Work out the finished part from the listing and answer in its coordinate system (mm). A direction names the side the tool comes from. Round coordinates to 2 decimals unless told otherwise and drop trailing zeros. Loops run counter-clockwise (first coordinate to the right, second up) from the corner with the lowest first, then second, coordinate; pieces in that order, holes last.
Autodesk Inventor part; units mm, degrees
ref_plane "YZ Plane" through (0, 0, 0) normal (1, 0, 0) x (0, 1, 0)
ref_plane "XZ Plane" through (0, 0, 0) normal (0, 1, 0) x (-1, 0, 0)
ref_plane "XY Plane" through (0, 0, 0) normal (0, 0, 1) x (1, 0, 0)
sketch "Szkic1" plane through (0, 0, 0) normal (0, 0, 1) x (1, 0, 0)
  line L0 (0, 0) -> (20, 0)
  line L1 (0, 0) -> (-20, 0)
  line L2 (-20, 0) -> (-20, 20)
  line L3 (-20, 0) -> (0, 0) construction
  line L4 (-20, 20) -> (20, 20)
  line L5 (20, 20) -> (20, 0)
  line L6 (-20, 0) -> (-20, 88)
  line L7 (-20, 88) -> (20, 88)
  line L8 (20, 88) -> (20, 20)
  line L9 (20, 88) -> (20, 93)
  line L10 (20, 93) -> (-20, 93)
  line L11 (-20, 93) -> (-20, 88)
  line L12 (0, 93) -> (35, 93)
  line L13 (35, 93) -> (40, 93)
  line L14 (0, 93) -> (-35, 93)
  line L15 (-35, 93) -> (-40, 93)
  line L16 (-40, 93) -> (-40, 103)
  line L17 (-40, 103) -> (40, 103)
  line L18 (40, 103) -> (40, 93)
  line L19 (-35, 93) -> (-35, 103)
  line L20 (35, 93) -> (35, 103)
  circle A0 centre (-35, 103) radius 1.5
  circle A1 centre (-35, 93) radius 1.5
  circle A2 centre (35, 103) radius 1.5
  circle A3 centre (35, 93) radius 1.5
  line L21 (40, 93) -> (40, 83)
  line L22 (40, 83) -> (20, 83)
  line L23 (-40, 93) -> (-40, 83)
  line L24 (-40, 83) -> (-20, 83)
  line L25 (-40, 103) -> (-40, 183)
  line L26 (40, 103) -> (40, 183)
  line L27 (40, 183) -> (-40, 183)
  dimension "d0" = 20
  dimension "d1" = 20
  dimension "d2" = 20
  dimension "d3" = 90
  dimension "d4" = 88
  dimension "d5" = 5
  dimension "d6" = 35
  dimension "d7" = 5
  dimension "d8" = 35
  dimension "d9" = 5
  dimension "d10" = 10
  dimension "d11" = 3
  dimension "d12" = 3
  dimension "d13" = 3
  dimension "d14" = 3
  dimension "d15" = 10
  dimension "d16" = 10
  dimension "d17" = 80
  dimension "d18" = 80
extrude "Wyciągnięcie proste1" add sketch "Szkic1" along normal blind 8
sketch "Szkic2" plane through (0, 0, 8) normal (0, 0, 1) x (1, 0, 0)
  circle A0 centre (-35, 103) radius 1.5
  circle A1 centre (-35, 93) radius 1.5
  circle A2 centre (35, 103) radius 1.5
  circle A3 centre (35, 93) radius 1.5
  line L0 (-35, 103) -> (35, 103)
  line L1 (-35, 93) -> (35, 93)
  line L2 (-35, 103) -> (-20, 103)
  line L3 (-20, 103) -> (-20, 93)
  line L4 (35, 103) -> (20, 103)
  line L5 (20, 103) -> (20, 93)
  circle A4 centre (-20, 103) radius 2
  circle A5 centre (-20, 93) radius 2
  circle A6 centre (20, 103) radius 2
  circle A7 centre (20, 93) radius 2
  line L6 (40, 83) -> (40, 183)
  line L7 (40, 183) -> (-40, 183)
  line L8 (-40, 183) -> (-40, 83)
  line L9 (-40, 83) -> (-20, 83)
  line L10 (-20, 83) -> (-20, 0)
  line L11 (-20, 0) -> (20, 0)
  line L12 (20, 0) -> (20, 83)
  line L13 (20, 83) -> (40, 83)
  line L14 (-20, 0) -> (20, 0)
  line L15 (-20, 0) -> (-20, 10)
  line L16 (-20, 83) -> (-20, 0)
  line L17 (-20, 10) -> (20, 10)
  line L18 (-20, 10) -> (-10, 10)
  line L19 (20, 10) -> (10, 10)
  circle A8 centre (-10, 10) radius 3
  circle A9 centre (10, 10) radius 3
  point P0 (0, 0)
  dimension "d21" = 15
  dimension "d22" = 15
  dimension "d23" = 4
  dimension "d24" = 4
  dimension "d25" = 4
  dimension "d26" = 4
  dimension "d27" = 10
  dimension "d28" = 10
  dimension "d29" = 10
  dimension "d30" = 6
  dimension "d31" = 6
hole "Otwór1" at (-20, 103, 8) at (-20, 93, 8) at (20, 103, 8) at (20, 93, 8) at (-35, 103, 8) at (-35, 93, 8) at (35, 103, 8) at (35, 93, 8) direction (0, 0, -1) diameter 4 end through all
sketch "Szkic3" plane through (0, 0, 8) normal (0, 0, 1) x (1, 0, 0)
  circle A0 centre (-10, 10) radius 3
  circle A1 centre (10, 10) radius 3
  point P0 (0, 0)
hole "Otwór2" at (-10, 10, 8) at (10, 10, 8) direction (0, 0, -1) diameter 6 end through all
fillet "Zaokrąglenie1" radius 20 2 edges at (20, 83, 4) (-20, 83, 4)
sketch "Szkic4" plane through (0, 0, 8) normal (0, 0, 1) x (1, 0, 0)
  line L0 (40, 183) -> (-40, 183)
  line L1 (40, 83) -> (40, 183)
  line L2 (40, 183) -> (-40, 183)
  line L3 (-40, 183) -> (-40, 333)
  line L4 (-40, 333) -> (0, 333)
  line L5 (40, 183) -> (40, 233)
  line L6 (40, 233) -> (0, 333)
  point P0 (0, 0)
  dimension "d47" = 150
  dimension "d50" = 50
extrude "Wyciągnięcie proste2" add sketch "Szkic4" against normal up to surface (8 mm away)
sketch "Szkic5" plane through (0, 0, 8) normal (0, 0, 1) x (1, 0, 0)
  line L0 (0, 333) -> (-40, 333)
  line L1 (-40, 333) -> (-40, 83)
  line L2 (-40, 333) -> (-40, 308)
  line L3 (-40, 308) -> (-17, 308)
  circle A0 centre (-17, 308) radius 13.5
  point P0 (0, 0)
  dimension "d51" = 25
  dimension "d52" = 23
  dimension "d53" = 27
extrude "Wyciągnięcie proste4" cut sketch "Szkic5" against normal up to next
sketch "Szkic7" plane through (0, 0, 0) normal (0, 0, -1) x (-1, 0, 0)
  line L0 (0, 333) -> (-40, 233)
  line L1 (0, 333) -> (40, 333)
  line L2 (0, 333) -> (-10, 333)
  line L3 (-10, 333) -> (-40, 233)
  point P0 (0, 0)
  dimension "d59" = 10
extrude "Wyciągnięcie proste5" add sketch "Szkic7" against normal blind 8
sketch "Szkic9" plane through (0, 0, 0) normal (0, 0, -1) x (-1, 0, 0)
  circle A0 centre (17, 308) radius 15
  line L0 (42, 333) -> (-8, 333)
  line L1 (-8, 333) -> (-23, 283)
  line L2 (-23, 283) -> (42, 283)
  line L3 (42, 283) -> (42, 333)
  line L4 (-10, 333) -> (40, 333)
  line L5 (40, 83) -> (40, 333)
  circle A1 centre (0, 325) radius 2
  circle A2 centre (34, 325) radius 2
  circle A3 centre (0, 291) radius 2
  circle A4 centre (34, 291) radius 2
  circle A5 centre (17, 308) radius 13.5
  point P0 (0, 0)
  point P1 (42, 283)
  dimension "d62" = 4
  dimension "d63" = 4
  dimension "d64" = 4
  dimension "d65" = 4
extrude "Wyciągnięcie proste6" cut sketch "Szkic9" against normal up to next contours A1 | A2 | A3 | A4
thread "Gwint1"
thread "Gwint2"
thread "Gwint3"
thread "Gwint4"
sketch "Szkic11" plane through (0, 0, 8) normal (0, 0, 1) x (1, 0, 0)
  line L0 (-40, 333) -> (-40, 83)
  line L1 (10, 333) -> (-40, 333)
  line L2 (-40, 333) -> (-40, 243)
  line L3 (-40, 83) -> (-40, 333)
  line L4 (-40, 333) -> (50, 333) construction
  line L5 (-40, 243) -> (0, 243)
  line L6 (0, 243) -> (0, 163)
  line L7 (0, 163) -> (-40, 163)
  line L8 (-40, 243) -> (-20, 243)
  line L9 (-20, 243) -> (-20, 163)
  line L10 (-20, 163) -> (-20, 203)
  line L11 (-20, 243) -> (-20, 223)
  line L12 (-20, 203) -> (-20, 213)
  line L13 (-20, 243) -> (-20, 253)
  circle A0 centre (-20, 213) radius 4.5
  circle A1 centre (-20, 253) radius 4.5
  point P0 (0, 0)
  dimension "d76" = 90
  dimension "d77" = 90
  dimension "d78" = 40
  dimension "d79" = 80
  dimension "d80" = 20
  dimension "d81" = 40
  dimension "d82" = 20
  dimension "d113" = 10
  dimension "d114" = 10
  dimension "d115" = 9
  dimension "d116" = 9
extrude "Wyciągnięcie proste7" cut sketch "Szkic11" against normal up to next contours A1 | A0 L9 | L9 A0
sketch "Szkic12" plane through (0, 0, 8) normal (0, 0, 1) x (1, 0, 0)
  line L0 (40, 233) -> (10, 333)
  line L1 (10, 333) -> (-40, 333)
  line L2 (-40, 333) -> (-40, 83)
  line L3 (40, 83) -> (40, 233)
  arc A0 (-20, 63) -> (-40, 83) centre (-40, 63) ccw
  arc A1 (40, 83) -> (20, 63) centre (40, 63) ccw
  line L4 (-40, 283) -> (20, 283)
  line L5 (20, 283) -> (20, 223)
  line L6 (-40, 223) -> (20, 223)
  line L7 (-40, 223) -> (-40, 283)
  circle A2 centre (0, 291) radius 2
  circle A3 centre (0, 325) radius 2
  circle A4 centre (-34, 325) radius 2
  circle A5 centre (-34, 291) radius 2
  circle A6 centre (-17, 308) radius 13.5
  circle A7 centre (-10, 10) radius 3
  circle A8 centre (10, 10) radius 3
  circle A9 centre (35, 103) radius 2
  circle A10 centre (-35, 103) radius 2
  circle A11 centre (20, 103) radius 2
  circle A12 centre (-20, 103) radius 2
  circle A13 centre (-20, 93) radius 2
  circle A14 centre (20, 93) radius 2
  circle A15 centre (-35, 93) radius 2
  circle A16 centre (35, 93) radius 2
  line L8 (-20, 63) -> (-20, 0)
  line L9 (-20, 0) -> (20, 0)
  line L10 (20, 0) -> (20, 63)
  arc A17 (40, 83) -> (20, 63) centre (40, 63) ccw
  line L11 (40, 83) -> (40, 233)
  line L12 (40, 233) -> (10, 333)
  line L13 (10, 333) -> (-40, 333)
  line L14 (-40, 333) -> (-40, 83)
  arc A18 (-20, 63) -> (-40, 83) centre (-40, 63) ccw
  line L15 (-35, 258) -> (-35, 253)
  line L16 (-5, 278) -> (-5, 273)
  line L17 (-35, 228) -> (-35, 233)
  line L18 (-5, 228) -> (-5, 233)
  circle A19 centre (-35, 233) radius 2.5
  circle A20 centre (-5, 233) radius 2.5
  circle A21 centre (-5, 273) radius 2.5
  circle A22 centre (-35, 253) radius 2.5
  line L19 (-37.5, 248) -> (-37.5, 258)
  arc A23 (-32.5, 258) -> (-37.5, 258) centre (-35, 258) ccw
  line L20 (-32.5, 258) -> (-32.5, 248)
  arc A24 (-37.5, 248) -> (-32.5, 248) centre (-35, 248) ccw
  line L21 (-2.5, 238) -> (-2.5, 228)
  arc A25 (-7.5, 228) -> (-2.5, 228) centre (-5, 228) ccw
  line L22 (-7.5, 228) -> (-7.5, 238)
  arc A26 (-2.5, 238) -> (-7.5, 238) centre (-5, 238) ccw
  line L23 (-37.5, 228) -> (-37.5, 238)
  arc A27 (-32.5, 238) -> (-37.5, 238) centre (-35, 238) ccw
  line L24 (-32.5, 238) -> (-32.5, 228)
  arc A28 (-37.5, 228) -> (-32.5, 228) centre (-35, 228) ccw
  line L25 (-2.5, 278) -> (-2.5, 268)
  arc A29 (-7.5, 268) -> (-2.5, 268) centre (-5, 268) ccw
  line L26 (-7.5, 268) -> (-7.5, 278)
  arc A30 (-2.5, 278) -> (-7.5, 278) centre (-5, 278) ccw
  line L27 (-30, 248) -> (-30, 258)
  arc A31 (-10, 258) -> (-30, 258) centre (-20, 258) ccw
  line L28 (-10, 258) -> (-10, 248)
  arc A32 (-30, 248) -> (-10, 248) centre (-20, 248) ccw
  line L29 (-40, 223) -> (-40, 283)
  line L30 (-40, 223) -> (20, 223)
  line L31 (20, 283) -> (20, 223)
  line L32 (-40, 283) -> (20, 283)
  line L33 (-35, 278) -> (-35, 283)
  line L34 (-5, 278) -> (-5, 283)
  line L35 (-35, 228) -> (-35, 223)
  line L36 (-5, 228) -> (-5, 223)
  line L37 (10, 333) -> (-40, 333)
  line L38 (-40, 333) -> (-40, 283)
  line L39 (-40, 83) -> (-40, 333)
  point P0 (0, 0)
  point P1 (30, 43)
  point P2 (-35, 248)
  point P3 (-5, 268)
  point P4 (-5, 238)
  point P5 (-35, 238)
  dimension "d87" = 5
  dimension "d88" = 5
  dimension "d89" = 5
  dimension "d90" = 5
  dimension "d91" = 5
  dimension "d92" = 5
  dimension "d93" = 5
  dimension "d94" = 5
  dimension "d118" = 50
extrude "Wyciągnięcie proste8" cut sketch "Szkic12" against normal up to next contours A19 | A21 | A20 | A22
thread "Gwint9"
thread "Gwint10"
thread "Gwint11"
thread "Gwint12"
thread "Gwint13"
thread "Gwint14"
thread "Gwint15"
thread "Gwint16"
properties part number "Wspornik pionowy osi Y - prawa strona"
1. Given pin 1 (3 mm diameter, centred on x = -34, y = 291, fed in from +Z); pin 2 (5 mm diameter, centred on x = 20, y = 103, fed in from +Z), each flat-ended and moving along its own axis, determine where each tip first touches the part or whether it passes through.
Answer key:
pin 1: passes through
pin 2: stops at z = 8
2. Find section A-A (y = 213). Write down the section's boundary in (x, z).
Answer key:
outline: (-40, 0) - (-24.5, 0) - (-24.5, 8) - (-40, 8) - close; (-15.5, 0) - (40, 0) - (40, 8) - (-15.5, 8) - close
3. Which of the six approach directions +Z, -Z, +X, -X, +Y, -Y give full straight-line access (tool end or side, diameter ignored) to faces 1 (the face through (-20, 31, 4)), 2 (the face through (20, 32, 4)), 3 (the face through (-18.757, 321.385, 4.056))?
Answer key:
face 1: +Z, -Z, -X, -Y
face 2: +Z, -Z, +X, -Y
face 3: +Z, -Z
4. Find section C-C (y = 10). Write down the section's boundary in (x, z).
Answer key:
outline: (-20, 0) - (-13, 0) - (-13, 8) - (-20, 8) - close; (-7, 0) - (7, 0) - (7, 8) - (-7, 8) - close; (13, 0) - (20, 0) - (20, 8) - (13, 8) - close
5. Determine the mould class of faces 4 (the face through (-20.98, 208.61, 4.06)), 5 (the face through (-25.703, 76.986, 4.056)), 6 (the face through (1, 169, 8)), 7 (the face through (-15, 333, 4)) for opening direction Y: +Y half, -Y half, draft (parallel to the pull), parting line (faces both ways), or undercut.
Answer key:
face 4: undercut
face 5: -Y half
face 6: draft
face 7: +Y half
6. Find section B-B (z = 3.75). Give the number of separate pieces and of enclosed holes in the cut face, then the cut area to 3 significant figures.
Answer key:
separate pieces: 1
enclosed holes: 21
area: 21,000 mm2
7. Consider probe 1 along X at (y, z) = (213, 4); probe 2 along Y at (x, z) = (-17, 4.5); probe 3 along Y at (x, z) = (-5, 4.5). Determine where each line is inside the solid, lowest interval first.
Answer key:
probe 1: x = -40 to -24.5, -15.5 to 40
probe 2: y = 0 to 209.65, 216.35 to 249.65, 256.35 to 294.5, 321.5 to 333
probe 3: y = 0 to 230.5, 235.5 to 270.5, 275.5 to 301.82, 314.18 to 333
